Can you work these out from the model? Positions are in its coordinate system, mm. A direction names the side the tool comes from. Coordinates: 2 decimals unless noted, no trailing zeros. Loops run counter-clockwise (first coordinate to the right, second up) from the corner with the lowest first, then second, coordinate; pieces in that order, holes last.
```python
from build123d import *

# Parameters (mm, degrees)
F1_DEPTH = 6
F2_R     = 1.5
F3_DEPTH = 25


with BuildPart() as f1:
    # F0 (on Top) → F1 (new body, symmetric)
    with BuildSketch(Plane.XY):
        Polygon((47.5, 20.5), (47.5, 28.5), (-47.5, 28.5), (-47.5, -28.5), (47.5, -28.5), (47.5, 4.5), (6.5, 4.5), (6.5, 20.5), align=None)
    extrude(amount=F1_DEPTH, both=True)

    # F2 (on face) → F3 (cut)
    with BuildSketch(Plane.XY.offset(6)):
        with Locations((-43, -20.5)):
            Circle(F2_R)
        with Locations((-27, -20.5)):
            Circle(F2_R)
        with Locations((26.5, -5.5)):
            Circle(F2_R)
        with Locations((42.5, -5.5)):
            Circle(F2_R)
        with Locations((42.5, 24.5)):
            Circle(F2_R)
        with Locations((26.5, 24.5)):
            Circle(F2_R)
    extrude(amount=-F3_DEPTH, mode=Mode.SUBTRACT)


solid = f1.part
```
Item 1: We'd pull the mould along X, two halves only. Please class faces 1 (the face through (-1, -28.5, 0)), 2 (the face through (6.5, 12, 0)), 3 (the face through (-28.11, -19.49, 0.08)): +X half, -X half, draft (parallel to the pull), parting line (faces both ways), or undercut.
Results are:
face 1: draft
face 2: +X half
face 3: undercut
Item 2: Suppose I cut it at D-D, the plane z = -2.5. Please give me the cut outline in (x, y).
Results are:
outline: (-47.5, -28.5) - (47.5, -28.5) - (47.5, 4.5) - (6.5, 4.5) - (6.5, 20.5) - (47.5, 20.5) - (47.5, 28.5) - (-47.5, 28.5) - close; hole circle Ø3 at (-43, -20.5); hole circle Ø3 at (-27, -20.5); hole circle Ø3 at (26.5, -5.5); hole circle Ø3 at (26.5, 24.5); hole circle Ø3 at (42.5, -5.5); hole circle Ø3 at (42.5, 24.5)
Item 3: On a 3-axis mill with a long thin cutter (end or side, diameter ignored), from which of +Z, -Z, +X, -X, +Y, -Y can I reach the whole of each face in a straight line? I mean faces 4 (the face through (47.5, -12, 0)), 5 (the face through (27, 20.5, 0)). Say none if no direction works.
Results are:
face 4: +Z, -Z, +X, +Y, -Y
face 5: +Z, -Z, +X
Item 4: Suppose I cut it at A-A, the plane x = 26.5. Please give me the cut outline in (y, z), plus the area to 3 significant figures.
Results are:
outline: (-28.5, -6) - (-7, -6) - (-7, 6) - (-28.5, 6) - close; (-4, -6) - (4.5, -6) - (4.5, 6) - (-4, 6) - close; (20.5, -6) - (23, -6) - (23, 6) - (20.5, 6) - close; (26, -6) - (28.5, -6) - (28.5, 6) - (26, 6) - close
area: 420 mm2
Item 5: Suppose I cut it at B-B, the plane y = -20.5. Please give me the cut outline in (x, z), plus the area to 3 significant figures.
Results are:
outline: (-47.5, -6) - (-44.5, -6) - (-44.5, 6) - (-47.5, 6) - close; (-41.5, -6) - (-28.5, -6) - (-28.5, 6) - (-41.5, 6) - close; (-25.5, -6) - (47.5, -6) - (47.5, 6) - (-25.5, 6) - close
area: 1,070 mm2
Item 6: Suppose I cut it at C-C, the plane x = -27. Please give me the cut outline in (y, z).
Results are:
outline: (-28.5, -6) - (-22, -6) - (-22, 6) - (-28.5, 6) - close; (-19, -6) - (28.5, -6) - (28.5, 6) - (-19, 6) - close
Item 7: I'm going to push a flat-ended pin straight in: P1, Ø6, axis at y = 11.5, z = 0.5, coming from the +X side. Where does the tip first touch, or does it pass through?
Results are:
P1: stops at x = 6.5
Item 8: I need wall thicknesses on line 1 along Y through (x, z) = (26.5, 0); line 2 along X through (y, z) = (-5, 0.75); line 3 along Y through (x, z) = (42, 0). Which ranges of each line are inside material? Lowest first, please.
Results are:
line 1: y = -28.5 to -7, -4 to 4.5, 20.5 to 23, 26 to 28.5
line 2: x = -47.5 to 25.09, 27.91 to 41.09, 43.91 to 47.5
line 3: y = -28.5 to -6.91, -4.09 to 4.5, 20.5 to 23.09, 25.91 to 28.5
